Read the model definition and answer for the solid it produces. Units are mm, in the model's axes. A direction names the side the tool comes from. Give positions to 0.01 mm unless a question says otherwise; leave off trailing zeros. Write each loop counter-clockwise with the first axis right and the second up, starting at its lowest first coordinate (ties: lowest second). Pieces come first, ordered by that corner, then holes.
```python
from build123d import *

# Parameters (mm, degrees)
SKETCH1_W           = 5
SKETCH1_H           = 40
BOSS_EXTRUDE1_DEPTH = 3
FILLET1_R           = 2


with BuildPart() as part:
    # Sketch1 → Boss-Extrude1 (new body)
    with BuildSketch(Plane.XY):
        with Locations((2.5, 20)):
            Rectangle(SKETCH1_W, SKETCH1_H)
        with BuildLine():
            Line((3.55, 37.5), (3.55, 2.5))
            ThreePointArc((3.55, 2.5), (2.5, 1.45), (1.45, 2.5))
            Line((1.45, 2.5), (1.45, 37.5))
            ThreePointArc((1.45, 37.5), (2.5, 38.55), (3.55, 37.5))
        make_face(mode=Mode.SUBTRACT)
    extrude(amount=BOSS_EXTRUDE1_DEPTH)

    # Fillet1
    fillet1_edges = [part.edges().sort_by_distance(p)[0] for p in [
        (0, 40, 1.5),
        (5, 40, 1.5),
        (5, 0, 1.5),
        (0, 0, 1.5),
    ]]
    fillet(fillet1_edges, radius=FILLET1_R)


solid = part.part
```
Item 1: Section A-A (x = 2.5) is taken. Write down the section's boundary in (y, z), and give its area (3 significant figures).
Result set:
outline: (0, 0) - (1.45, 0) - (1.45, 3) - (0, 3) - close; (38.55, 0) - (40, 0) - (40, 3) - (38.55, 3) - close
area: 8.70 mm2
Item 2: Which of the six approach directions +Z, -Z, +X, -X, +Y, -Y give full straight-line access (tool end or side, diameter ignored) to faces 1 (the cylindrical face through (2.52, 1.45, 1.48)), 2 (the flat face through (2.5, 40, 1.5))?
Result set:
face 1: +Z, -Z
face 2: +Z, -Z, +X, -X, +Y
Item 3: Section C-C (y = 9.5) is taken. Write down the section's boundary in (x, z), and give its area (3 significant figures).
Result set:
outline: (0, 0) - (1.45, 0) - (1.45, 3) - (0, 3) - close; (3.55, 0) - (5, 0) - (5, 3) - (3.55, 3) - close
area: 8.70 mm2
Item 4: Find the intervals of material crossed by line 1 along X through (y, z) = (9, 2.2); line 2 along Y through (x, z) = (3.4, 1.35), in increasing order.
Result set:
line 1: x = 0 to 1.45, 3.55 to 5
line 2: y = 0.04 to 1.96, 38.04 to 39.96
Item 5: Section D-D (x = 0.4) is taken. Write down the section's boundary in (y, z).
Result set:
outline: (0.8, 0) - (39.2, 0) - (39.2, 3) - (0.8, 3) - close
Item 6: Section B-B (z = 1.85) is taken. Write down the section's boundary in (x, y), and give its area (3 significant figures).
Result set:
outline: (0, 2) arc R2 ccw to (2, 0) - (3, 0) arc R2 ccw to (5, 2) - (5, 38) arc R2 ccw to (3, 40) - (2, 40) arc R2 ccw to (0, 38) - close; hole (1.45, 2.5) arc R1.05 ccw to (3.55, 2.5) - (3.55, 37.5) arc R1.05 ccw to (1.45, 37.5) - close
area: 120 mm2
